```python
from build123d import *

# Parameters (mm, degrees)
CIRPATTERN2_COUNT  = 16
FILLET1_R          = 5
SKETCH7_R          = 9
CUT_EXTRUDE1_DEPTH = 198.404407246
SKETCH3_R          = 6.5
CUT_EXTRUDE2_DEPTH = 198.404407246


with BuildPart() as part:
    # Sketch1 → Revolve1 (revolve)
    with BuildSketch(Plane.XY, mode=Mode.PRIVATE) as revolve1_sk:
        Polygon((24, 137.5), (24, 99.5), (34, 99.5), (34, 60), (0, 60), (0, 137.5), align=None)
    revolve(revolve1_sk.sketch.rotate(Axis((0, 0, 0), (1, 0, 0)), 90), axis=Axis((0, 0, 0), (1, 0, 0)))

    # Sketch6 → M10 Tapped Hole1 (revolve, cut)
    with BuildSketch(Plane(origin=(0, -110.418238983, 63.75), x_dir=(0, 0, 1), z_dir=(0, 1, 0))):
        Polygon((0, 0), (0, 41.053657631), (4.25, 38.5), (4.25, 0.775), (5.025, 0), align=None)
    m10_tapped_hole1 = revolve(axis=Axis((-6.35, -110.418238983, 63.75), (1, 0, 0)), mode=Mode.SUBTRACT)

    # CirPattern2: M10 Tapped Hole1 ×16 about axis
    cirpattern2_axis = Axis((0, 0, 0), (1, 0, 0))
    for i in range(1, CIRPATTERN2_COUNT):
        add(m10_tapped_hole1.rotate(cirpattern2_axis, i * 360 / CIRPATTERN2_COUNT), mode=Mode.SUBTRACT)

    # Fillet1
    fillet1_edges = [part.edges().sort_by_distance(p)[0] for p in [
        (24, 0, -99.5),
    ]]
    fillet(fillet1_edges, radius=FILLET1_R)

    # Sketch7 → Cut-Extrude1 (cut, through all)
    with BuildSketch(Plane.ZY):
        with Locations((73.5, 0)):
            Circle(SKETCH7_R)
        with Locations((-36.75, -63.652867178)):
            Circle(SKETCH7_R)
        with Locations((-36.75, 63.652867178)):
            Circle(SKETCH7_R)
    extrude(amount=-CUT_EXTRUDE1_DEPTH, mode=Mode.SUBTRACT)

    # Sketch3 → Cut-Extrude2 (cut, through all)
    with BuildSketch(Plane.ZY):
        with Locations((0, 80)):
            Circle(SKETCH3_R)
        with Locations((40, 69.282032303)):
            Circle(SKETCH3_R)
        with Locations((69.282032303, 40)):
            Circle(SKETCH3_R)
        with Locations((69.282032303, -40)):
            Circle(SKETCH3_R)
        with Locations((40, -69.282032303)):
            Circle(SKETCH3_R)
        with Locations((0, -80)):
            Circle(SKETCH3_R)
        with Locations((-69.282032303, -40)):
            Circle(SKETCH3_R)
        with Locations((-80, 0)):
            Circle(SKETCH3_R)
        with Locations((-69.282032303, 40)):
            Circle(SKETCH3_R)
    extrude(amount=-CUT_EXTRUDE2_DEPTH, mode=Mode.SUBTRACT)


solid = part.part
```
Could you check a few things on this model? Use its own coordinates, in mm. Give positions to 0.01 mm unless a question says otherwise; leave off trailing zeros. Write each question's results on one line, items separated by ' | '.
1. If we mould it in two halves opening along Y, with no side actions, what happens to faces 1 (the cylindrical face through (12.225, 111.695, -67.804)), 2 (the flat face through (0, 29, -59))? For each: released by +Y, released by -Y, zero draft, split by the parting line, or undercut.
Check sheet entries:
face 1: undercut | face 2: zero draft
2. I want a section at A-A, the plane x = 13.5. Count the separate pieces of the cut face and the enclosed holes in it, then the cut area to 3 significant figures.
Check sheet entries:
separate pieces: 1 | enclosed holes: 29 | area: 45,200 mm²
3. Will these pins go through, and if not, where does the flat tip stop? pin 1 Ø7.5 at (y, z) = (77.62, -101.15) entering from +X; pin 2 Ø1.5 at (x, z) = (17, -48) entering from +Y; pin 3 Ø6 at (x, z) = (28, -58.5) entering from +Y; pin 4 Ø10 at (x, z) = (17, -19) entering from +Y.
Check sheet entries:
pin 1: passes through | pin 2: stops at y = 129.13 | pin 3: stops at y = 83.41 | pin 4: stops at y = 136.79
4. I need wall thicknesses on L1, parallel to Y at x = 15.5, z = -38; L2, parallel to Z at x = 8, y = 74; L3, parallel to Y at x = 7.5, z = -14.5. Which ranges of each line are inside material? Lowest first, please.
Check sheet entries:
L1: y = -132.14 to -72.57, -54.74 to -46.43, 46.43 to 54.74, 72.57 to 132.14 | L2: z = -115.89 to -103.38, -98.92 to -2.5, 2.5 to 35.53, 44.47 to 115.89 | L3: y = -136.73 to -58.22, 58.22 to 122.74, 130.08 to 136.73
